from build123d import *

# Parameters (mm, degrees)
SKETCH1_R               = 6
BOSS_EXTRUDE1_DEPTH     = 24.3
SKETCH8_R               = 6.35
BOSS_EXTRUDE5_DEPTH     = 2.5
BOSS_EXTRUDE6_DEPTH     = 2.5
CIRPATTERN1_COUNT       = 11
SKETCH10_R              = 6
BOSS_EXTRUDE7_DEPTH     = 3
CUT_EXTRUDE3_DEPTH      = 33.398962536
CUT_EXTRUDE3_DEPTH_BACK = 33.398962536
SKETCH11_R              = 5


with BuildPart() as part:
    # Sketch1 → Boss-Extrude1 (new body)
    with BuildSketch(Plane(origin=(0, 0, 0), x_dir=(1, 0, 0), z_dir=(0, 1, 0))):
        with Locations(Location((0, 0, 0), (0, 0, 270))):
            Circle(SKETCH1_R)
    extrude(amount=BOSS_EXTRUDE1_DEPTH)

    # Sketch8 → Boss-Extrude5 (add)
    with BuildSketch(Plane(origin=(0, 24.3, 0), x_dir=(-1, 0, 0), z_dir=(0, 1, 0))):
        with Locations(Location((0, 0, 0), (0, 0, 90))):
            Circle(SKETCH8_R)
    extrude(amount=BOSS_EXTRUDE5_DEPTH)

    # Sketch9 → Boss-Extrude6 (add)
    with BuildSketch(Plane(origin=(0, 26.8, 0), x_dir=(1, 0, 0), z_dir=(0, 1, 0))):
        Polygon((0.508, -9), (-0.508, -9), (-1.286124455, -6.096), (1.286124455, -6.096), align=None)
    boss_extrude6 = extrude(amount=-BOSS_EXTRUDE6_DEPTH)

    # CirPattern1: Boss-Extrude6 ×11 about axis
    cirpattern1_axis = Axis((0, 0, 0), (0, 1, 0))
    for i in range(1, CIRPATTERN1_COUNT):
        add(boss_extrude6.rotate(cirpattern1_axis, i * 360 / CIRPATTERN1_COUNT))

    # Sketch10 → Boss-Extrude7 (add)
    with BuildSketch(Plane(origin=(0, 26.8, 0), x_dir=(1, 0, 0), z_dir=(0, 1, 0))):
        with Locations(Location((0, 0, 0), (0, 0, 270))):
            Circle(SKETCH10_R)
    extrude(amount=BOSS_EXTRUDE7_DEPTH)

    # Sketch11 → Cut-Extrude3 (cut, two sides: drawn at the far end of the back side and taken through both)
    with BuildSketch(Plane(origin=(0, 29.8, 0), x_dir=(-1, 0, 0), z_dir=(0, 1, 0)).offset(-CUT_EXTRUDE3_DEPTH_BACK)):
        with Locations(Location((0, 0, 0), (0, 0, 90))):
            Circle(SKETCH11_R)
    extrude(amount=CUT_EXTRUDE3_DEPTH + CUT_EXTRUDE3_DEPTH_BACK, mode=Mode.SUBTRACT)


solid = part.part
Build history of the part. All positions in model axes, mm. A direction names the side the tool comes from. Round coordinates to 2 decimals unless told otherwise and drop trailing zeros. Write each loop counter-clockwise with the first axis right and the second up, starting at its lowest first coordinate (ties: lowest second). Pieces come first, ordered by that corner, then holes. Notation, with made-up numbers: M 1,-39.5 L 39,-39.5 A18 cw 39,-35.5 Z; hole C 36,77.25 d2. An arc over 180 degrees is marked long. Use CSV: the item, a comma, the result in double quotes.
1. Saw through at B-B (z = 0). Give the cut face in (x, y).
Reply:
outline,"M -7.16,24.3 L -6,24.3 L -6,0 L -5,0 L -5,29.8 L -6,29.8 L -6,26.8 L -7.16,26.8 Z; M 5,0 L 6,0 L 6,24.3 L 7.16,24.3 L 7.16,26.8 L 6,26.8 L 6,29.8 L 5,29.8 Z"
2. Saw through at D-D (z = -7.5). Give the cut face in (x, y), plus the area to 3 significant figures.
Reply:
outline,"M -3,24.3 L -1.27,24.3 L -1.27,26.8 L -3,26.8 Z; M 1.27,24.3 L 3,24.3 L 3,26.8 L 1.27,26.8 Z"
area,"8.65 mm²"
3. Flat gauge pins, fed straight in: pin 1 (8 mm diameter, centred on x = 5, y = 12, fed in from +Z); pin 2 (8 mm diameter, centred on y = 7, z = -4, fed in from +X); pin 3 (9 mm diameter, centred on x = 0, z = 0, fed in from -Y); pin 4 (2 mm diameter, centred on x = -7, z = -5.5, fed in from -Y). Where does each tip first touch, or does it go through?
Reply:
pin 1,"stops at z = 5.92"
pin 2,"stops at x = 6"
pin 3,"passes through"
pin 4,"stops at y = 24.3"
4. Saw through at A-A (x = 0). Give the cut face in (y, z).
Reply:
outline,"M 0,-6 L 24.3,-6 L 24.3,-6.35 L 26.8,-6.35 L 26.8,-6 L 29.8,-6 L 29.8,-5 L 0,-5 Z; M 0,5 L 29.8,5 L 29.8,6 L 26.8,6 L 26.8,9 L 24.3,9 L 24.3,6 L 0,6 Z"
5. Wall check: probe 1 along X at (y, z) = (21.75, 0); probe 2 along X at (y, z) = (15.5, -1.25); probe 3 along Y at (x, z) = (-6, 1). Give the ranges that are in metal, low to high. Write a range as from..to.
Reply:
probe 1,"x = -6..-5, 5..6"
probe 2,"x = -5.87..-4.84, 4.84..5.87"
probe 3,"y = 24.3..26.8"
6. Saw through at C-C (y = 23.75). Give the cut face in (x, z).
Reply:
outline,"C 0,0 d12; hole C 0,0 d10"
7. Tool access for faces 1 (the face through (6, 24.3, 2)), 2 (the face through (0.885, 25.568, 7.593)), 3 (the face through (7.39, 25.568, -1.957)), 4 (the face through (-1.31, 25.57, -7.57)): list every direction of +Z, -Z, +X, -X, +Y, -Y with a clear straight run to the whole face (end or side of a thin tool).
Reply:
face 1,"-Y"
face 2,"+Z, +Y, -Y"
face 3,"+X, +Y, -Y"
face 4,"-Z, +Y, -Y"
8. Two-plate mould, pull along X, no slides. Class faces 5 (the face through (5.78, 25.53, -2.63)), 6 (the face through (-4.804, 25.532, 4.153)), 7 (the face through (-6.286, 25.532, 0.896)): +X half, -X half, draft (parallel to the pull), parting line (faces both ways), or undercut.
Reply:
face 5,"+X half"
face 6,"undercut"
face 7,"-X half"
